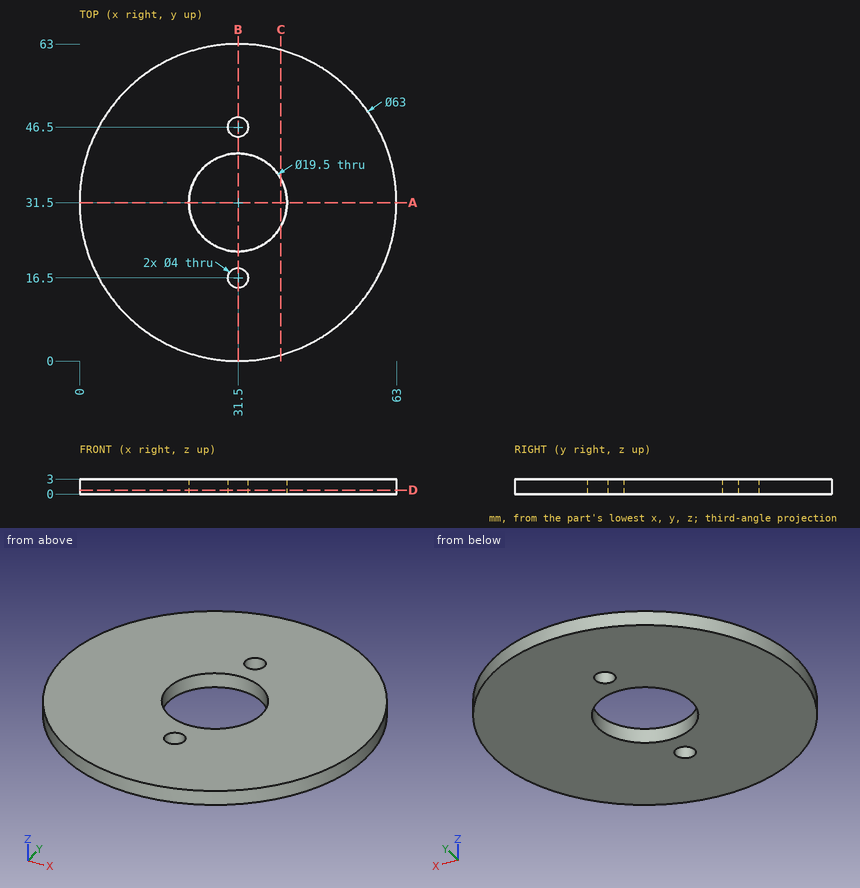
Geometry: see drawing. Coordinates: mm, zero at the bounding-box minimum. Round coordinates to 2 decimals unless told otherwise and drop trailing zeros. Write each loop counter-clockwise with the first axis right and the second up, starting at its lowest first coordinate (ties: lowest second). Pieces come first, ordered by that corner, then holes. Notation, with made-up numbers: M 49.5,67.5 L 67.5,67.5 A22 ccw 67.5,76.5 Z; hole C 54.25,17 d7. An arc over 180 degrees is marked long. Answer in a Markdown table with one row per item. Add a question column.
(1) Contact query for a flat-ended pin moving along its axis: pin 1 (1.5 mm diameter, centred on y = 41.5, z = 2, fed in from -X). Output: stop coordinate, or through.
(2) Cut plane B-B, the plane x = 31.5. Return the cut outline in (y, z).
(3) Cut plane A-A, the plane y = 31.5. Return the cut outline in (x, z).
(4) Cut plane D-D, the plane z = 0.8. Return the cut outline in (x, y).
(5) Cut plane C-C, the plane x = 40. Return the cut outline in (y, z), then the cut area to 3 significant figures.
(6) Ray query, L1, parallel to Y at x = 31.5, z = 1.25; L2, parallel to X at y = 17, z = 0.6; L3, parallel to X at y = 46.5, z = 1.45. Return the intervals inside material, ascending.
Established:
| question | item | result |
|---|---|---|
| 1 | pin 1 | x = 1.39 |
| 2 | outline | M 0,0 L 14.5,0 L 14.5,3 L 0,3 Z; M 18.5,0 L 21.75,0 L 21.75,3 L 18.5,3 Z; M 41.25,0 L 44.5,0 L 44.5,3 L 41.25,3 Z; M 48.5,0 L 63,0 L 63,3 L 48.5,3 Z |
| 3 | outline | M 0,0 L 21.75,0 L 21.75,3 L 0,3 Z; M 41.25,0 L 63,0 L 63,3 L 41.25,3 Z |
| 4 | outline | C 31.5,31.5 d63; hole C 31.5,31.5 d19.5; hole C 31.5,16.5 d4; hole C 31.5,46.5 d4 |
| 5 | outline | M 1.17,0 L 26.72,0 L 26.72,3 L 1.17,3 Z; M 36.28,0 L 61.83,0 L 61.83,3 L 36.28,3 Z |
| 5 | area | 153 mm² |
| 6 | L1 | 0 to 14.5, 18.5 to 21.75, 41.25 to 44.5, 48.5 to 63 |
| 6 | L2 | 3.54 to 29.56, 33.44 to 59.46 |
| 6 | L3 | 3.8 to 29.5, 33.5 to 59.2 |
